Here's how the part is built. I have some questions about the finished solid (model axes, mm). Face numbers are marked on the shaded views. A direction names the side the tool comes from. Coordinates: 2 decimals unless noted, no trailing zeros. Write each loop counter-clockwise with the first axis right and the second up, starting at its lowest first coordinate (ties: lowest second). Pieces come first, ordered by that corner, then holes. Notation, with made-up numbers: (61, 41) -> (117, 41) arc R12 cw to (117, 55) -> close; hole circle Ø11 at (28.25, 22). An arc over 180 degrees is marked (long way). Put each result on its own line as item: value. Start each with the question number.
Item 1: I want a section at D-D, the plane y = -52. List the corners of the cut face in (x, z) for me, then the cut area to 3 significant figures.
Item 2: I want a section at A-A, the plane z = 25. List the corners of the cut face in (x, y) for me.
Item 3: I want a section at C-C, the plane x = 47.5. List the corners of the cut face in (y, z) for me, then the cut area to 3 significant figures.
Item 4: If we mould it in two halves opening along X, with no side actions, what happens to the marked faces 1, 2, 3 and 4? For each: released by +X, released by -X, zero draft, split by the parting line, or undercut.
Item 5: On a 3-axis mill with a long thin cutter (end or side, diameter ignored), from which of +Z, -Z, +X, -X, +Y, -Y can I reach the whole of each face in a straight line? I mean the marked faces 5 and 6. Say none if no direction works.
Item 6: I need wall thicknesses on line 1 (Y direction, x = 66, z = 25); line 2 (X direction, y = 34.5, z = 2); line 3 (Y direction, x = -53.5, z = 23.5). Which ranges of each line are inside material? Lowest first, please. Write a range as [from, to].
Item 7: For pin 1 (0.6 mm diameter, centred on x = 22.5, y = -61, fed in from -Z); pin 2 (4 mm diameter, centred on x = -18.5, y = 23, fed in from +Z); pin 3 (1 mm diameter, centred on x = -51.5, y = 47, fed in from -Z), each with a flat end and sliding along its axis, tell me the tip position at first contact or that it passes through.
Item 8: I want a section at B-B, the plane y = 52. List the corners of the cut face in (x, z) for me.
Autodesk Inventor part; units mm, degrees
ref_plane "YZ Plane" through (0, 0, 0) normal (1, 0, 0) x (0, 1, 0)
ref_plane "XZ Plane" through (0, 0, 0) normal (0, 1, 0) x (-1, 0, 0)
ref_plane "XY Plane" through (0, 0, 0) normal (0, 0, 1) x (1, 0, 0)
sketch "스케치1" plane through (0, 0, 0) normal (0, 0, 1) x (1, 0, 0)
  line L0 (67, -62) -> (-67, -62)
  line L1 (-67, -62) -> (-67, 62)
  line L2 (-67, 62) -> (67, 62)
  line L3 (67, 62) -> (67, -62)
  line L4 (67, -62) -> (-67, 62) construction
  line L5 (-67, -62) -> (67, 62) construction
  point P0 (0, 0)
  dimension "d0" = 134
  dimension "d1" = 124
extrude "돌출1" add sketch "스케치1" along normal blind 28
shell "쉘1" thickness 1.2 removed faces 1 at (22.3333, 20.6667, 28)
sketch "스케치2" plane through (0, 0, 0) normal (0, 0, -1) x (-1, 0, 0)
  line L0 (59.4523, -61.8902) -> (-59.4523, -61.8902)
  line L1 (-59.4523, -61.8902) -> (-59.4523, -43.79)
  line L2 (-59.4523, -43.79) -> (59.4523, -43.79)
  line L3 (59.4523, -43.79) -> (59.4523, -61.8902)
  line L4 (59.4523, -61.8902) -> (-59.4523, -43.79) construction
  line L5 (-59.4523, -61.8902) -> (59.4523, -43.79) construction
  point P0 (0, 0)
  point P1 (0, -52.8401)
extrude "돌출2" cut sketch "스케치2" against normal blind 1.2
sketch "스케치3" plane through (0, 0, 0) normal (0, 0, -1) x (-1, 0, 0)
  line L0 (-31.3452, 31.9819) -> (-10.2317, 31.9819) construction
  line L1 (-10.2317, 31.9819) -> (-10.2317, 28.3571) construction
  line L2 (-10.2317, 28.3571) -> (-31.3452, 28.3571) construction
  line L3 (-31.3452, 28.3571) -> (-31.3452, 31.9819) construction
  spline S0 degree 2 poles (-23.1755, 23.6344) (-23.1755, 23.7476) (-23.1755, 23.9819) (-23.2078, 24.1597) knots 0 0 0 1 2 2 2
  line L4 (-23.2078, 24.1597) -> (-24.7432, 24.1597)
  spline S1 degree 2 poles (-24.7432, 24.1597) (-24.7432, 23.1981) (-25.325, 20.7657) (-26.7714, 20.7657) knots 0 0 0 1 2 2 2
  spline S2 degree 2 poles (-26.7714, 20.7657) (-28.3068, 20.8789) (-28.9129, 23.8122) (-28.9129, 25.4284) knots 0 0 0 1 2 2 2
  spline S3 degree 2 poles (-28.9129, 25.4284) (-28.9129, 25.5496) (-28.9129, 25.7758) (-28.9129, 25.8971) knots 0 0 0 1 2 2 2
  spline S4 degree 2 poles (-28.9129, 25.8971) (-28.9129, 27.0849) (-28.3472, 30.5597) (-26.828, 30.5597) knots 0 0 0 1 2 2 2
  spline S5 degree 2 poles (-26.828, 30.5597) (-25.4219, 30.5597) (-24.7432, 28.79) (-24.7432, 27.8364) knots 0 0 0 1 2 2 2
  line L5 (-24.7432, 27.8364) -> (-23.2078, 27.8364)
  spline S6 degree 2 poles (-23.2078, 27.8364) (-23.1755, 27.9819) (-23.1755, 28.1516) (-23.1755, 28.2162) knots 0 0 0 1 2 2 2
  spline S7 degree 2 poles (-23.1755, 28.2162) (-23.1755, 30.4142) (-25.325, 31.9819) (-26.6098, 31.9819) knots 0 0 0 1 2 2 2
  spline S8 degree 2 poles (-26.6098, 31.9819) (-29.4785, 31.893) (-30.4805, 27.4001) (-30.4805, 25.4284) knots 0 0 0 1 2 2 2
  spline S9 degree 2 poles (-30.4805, 25.4284) (-30.4805, 22.8829) (-29.131, 19.4567) (-26.6098, 19.3435) knots 0 0 0 1 2 2 2
  spline S10 degree 2 poles (-26.6098, 19.3435) (-24.7512, 19.3435) (-23.1755, 21.9536) (-23.1755, 23.6344) knots 0 0 0 1 2 2 2
  line L6 (-14.0765, 19.6021) -> (-14.0765, 31.6021)
  line L7 (-14.0765, 31.6021) -> (-15.6442, 31.6021)
  line L8 (-15.6442, 31.6021) -> (-15.6442, 26.7617)
  line L9 (-15.6442, 26.7617) -> (-19.927, 26.7617)
  line L10 (-19.927, 26.7617) -> (-19.927, 31.6021)
  line L11 (-19.927, 31.6021) -> (-21.4947, 31.6021)
  line L12 (-21.4947, 31.6021) -> (-21.4947, 19.6021)
  line L13 (-21.4947, 19.6021) -> (-19.927, 19.6021)
  line L14 (-19.927, 19.6021) -> (-19.927, 25.3395)
  line L15 (-19.927, 25.3395) -> (-15.6442, 25.3395)
  line L16 (-15.6442, 25.3395) -> (-15.6442, 19.6021)
  line L17 (-15.6442, 19.6021) -> (-14.0765, 19.6021)
  line L18 (-4.1371, 19.6021) -> (-7.4098, 31.6021)
  line L19 (-7.4098, 31.6021) -> (-9.4381, 31.6021)
  line L20 (-9.4381, 31.6021) -> (-12.7997, 19.6021)
  line L21 (-12.7997, 19.6021) -> (-11.1512, 19.6021)
  line L22 (-11.1512, 19.6021) -> (-10.2785, 22.9637)
  line L23 (-10.2785, 22.9637) -> (-6.6826, 22.9637)
  line L24 (-6.6826, 22.9637) -> (-5.8421, 19.6021)
  line L25 (-5.8421, 19.6021) -> (-4.1371, 19.6021)
  line L26 (-7.1189, 24.3859) -> (-9.8421, 24.3859)
  line L27 (-9.8421, 24.3859) -> (-8.4846, 30.0102)
  line L28 (-8.4846, 30.0102) -> (-7.1189, 24.3859)
  line L29 (3.4023, 30.1799) -> (3.4023, 31.6021)
  line L30 (3.4023, 31.6021) -> (-2.8603, 31.6021)
  line L31 (-2.8603, 31.6021) -> (-2.8603, 19.6021)
  line L32 (-2.8603, 19.6021) -> (3.2892, 19.6021)
  line L33 (3.2892, 19.6021) -> (3.2892, 21.0243)
  line L34 (3.2892, 21.0243) -> (-1.2927, 21.0243)
  line L35 (-1.2927, 21.0243) -> (-1.2927, 25.2263)
  line L36 (-1.2927, 25.2263) -> (3.0548, 25.2263)
  line L37 (3.0548, 25.2263) -> (3.0548, 26.6486)
  line L38 (3.0548, 26.6486) -> (-1.2927, 26.6486)
  line L39 (-1.2927, 26.6486) -> (-1.2927, 30.1799)
  line L40 (-1.2927, 30.1799) -> (3.4023, 30.1799)
  line L41 (12.2346, 19.6021) -> (12.2346, 31.6021)
  line L42 (12.2346, 31.6021) -> (10.6669, 31.6021)
  line L43 (10.6669, 31.6021) -> (10.6669, 26.7617)
  line L44 (10.6669, 26.7617) -> (6.3841, 26.7617)
  line L45 (6.3841, 26.7617) -> (6.3841, 31.6021)
  line L46 (6.3841, 31.6021) -> (4.8164, 31.6021)
  line L47 (4.8164, 31.6021) -> (4.8164, 19.6021)
  line L48 (4.8164, 19.6021) -> (6.3841, 19.6021)
  line L49 (6.3841, 19.6021) -> (6.3841, 25.3395)
  line L50 (6.3841, 25.3395) -> (10.6669, 25.3395)
  line L51 (10.6669, 25.3395) -> (10.6669, 19.6021)
  line L52 (10.6669, 19.6021) -> (12.2346, 19.6021)
  line L53 (26.1174, 31.6021) -> (24.5821, 31.6021)
  line L54 (24.5821, 31.6021) -> (22.6427, 21.7193)
  line L55 (22.6427, 21.7193) -> (20.7518, 31.6021)
  line L56 (20.7518, 31.6021) -> (19.0144, 31.6021)
  line L57 (19.0144, 31.6021) -> (16.9619, 21.7758)
  line L58 (16.9619, 21.7758) -> (15.1599, 31.6021)
  line L59 (15.1599, 31.6021) -> (13.5114, 31.6021)
  line L60 (13.5114, 31.6021) -> (16.0003, 19.6021)
  line L61 (16.0003, 19.6021) -> (17.8831, 19.6021)
  line L62 (17.8831, 19.6021) -> (19.8306, 29.687)
  line L63 (19.8306, 29.687) -> (21.7134, 19.6021)
  line L64 (21.7134, 19.6021) -> (23.5962, 19.6021)
  line L65 (23.5962, 19.6021) -> (26.1174, 31.6021)
  line L66 (29.1882, 19.6021) -> (29.1882, 31.6021)
  line L67 (29.1882, 31.6021) -> (27.6205, 31.6021)
  line L68 (27.6205, 31.6021) -> (27.6205, 19.6021)
  line L69 (27.6205, 19.6021) -> (29.1882, 19.6021)
  point P0 (0, 0)
  dimension "d0" = 134
  dimension "d1" = 124
extrude "돌출3" add sketch "스케치3" along normal blind 2
sketch "스케치5" plane through (-67, -62, 0) normal (0, -1, 0) x (1, 0, 0)
  line L0 (7.5477, 0) -> (126.4523, 0)
  line L1 (126.4523, 0) -> (7.5477, 0)
  line L2 (7.5477, 0) -> (7.5477, 15.3269)
  line L3 (7.5477, 15.3269) -> (126.4523, 15.3269)
  line L4 (126.4523, 15.3269) -> (126.4523, 0)
  point P0 (67, 0)
extrude "돌출5" cut sketch "스케치5" against normal blind 1.2
sketch "스케치6" plane through (67, -62, 0) normal (1, 0, 0) x (0, 0, -1)
  line L0 (-28, 0) -> (-28, 124) construction
  line L1 (-28, 124) -> (-25, 124) construction
  line L2 (0, 124) -> (-28, 124) construction
  line L3 (-25, 124) -> (-25, 114) construction
  circle A0 centre (-25, 114) radius 1.75
  line L4 (-28, 0) -> (-25, 0) construction
  line L5 (0, 0) -> (-28, 0) construction
  line L6 (-25, 0) -> (-25, 10) construction
  circle A1 centre (-25, 10) radius 1.75
  point P0 (0, 62)
  dimension "d13" = 3
  dimension "d14" = 10
  dimension "d15" = 3.5
  dimension "d16" = 3
  dimension "d17" = 10
  dimension "d18" = 3.5
extrude "돌출6" cut sketch "스케치6" against normal blind 200
properties part number "240621_뚜껑"
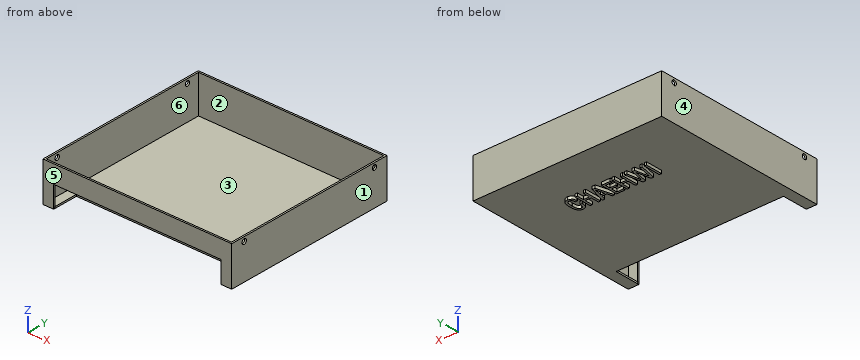
Calculated:
1. outline: (-67, 0) -> (-59.45, 0) -> (-59.45, 1.2) -> (-65.8, 1.2) -> (-65.8, 23.25) -> (-67, 23.25) -> close; (-67, 26.75) -> (-65.8, 26.75) -> (-65.8, 28) -> (-67, 28) -> close; (59.45, 0) -> (67, 0) -> (67, 23.25) -> (65.8, 23.25) -> (65.8, 1.2) -> (59.45, 1.2) -> close; (65.8, 26.75) -> (67, 26.75) -> (67, 28) -> (65.8, 28) -> close
1. area: 74.0 mm2
2. outline: (-67, -62) -> (67, -62) -> (67, -53.75) -> (65.8, -53.75) -> (65.8, -60.8) -> (-65.8, -60.8) -> (-65.8, -53.75) -> (-67, -53.75) -> close; (-67, -50.25) -> (-65.8, -50.25) -> (-65.8, 50.25) -> (-67, 50.25) -> close; (-67, 53.75) -> (-65.8, 53.75) -> (-65.8, 60.8) -> (65.8, 60.8) -> (65.8, 53.75) -> (67, 53.75) -> (67, 62) -> (-67, 62) -> close; (65.8, -50.25) -> (67, -50.25) -> (67, 50.25) -> (65.8, 50.25) -> close
3. outline: (-62, 15.33) -> (-60.8, 15.33) -> (-60.8, 28) -> (-62, 28) -> close; (-43.79, 0) -> (62, 0) -> (62, 28) -> (60.8, 28) -> (60.8, 1.2) -> (-43.79, 1.2) -> close
3. area: 174 mm2
4. face 1: released by +X
4. face 2: undercut
4. face 3: undercut
4. face 4: released by -X
5. face 5: +Z, -Z, +X, -X, -Y
5. face 6: +Z
6. line 1: y = [-62, -53.75], [-50.25, 50.25], [53.75, 62]
6. line 2: x = [-67, -65.8], [65.8, 67]
6. line 3: y = [-62, -60.8], [60.8, 62]
7. pin 1: stops at z = 15.33
7. pin 2: stops at z = 1.2
7. pin 3: stops at z = 0
8. outline: (-67, 0) -> (67, 0) -> (67, 23.25) -> (65.8, 23.25) -> (65.8, 1.2) -> (-65.8, 1.2) -> (-65.8, 23.25) -> (-67, 23.25) -> close; (-67, 26.75) -> (-65.8, 26.75) -> (-65.8, 28) -> (-67, 28) -> close; (65.8, 26.75) -> (67, 26.75) -> (67, 28) -> (65.8, 28) -> close
